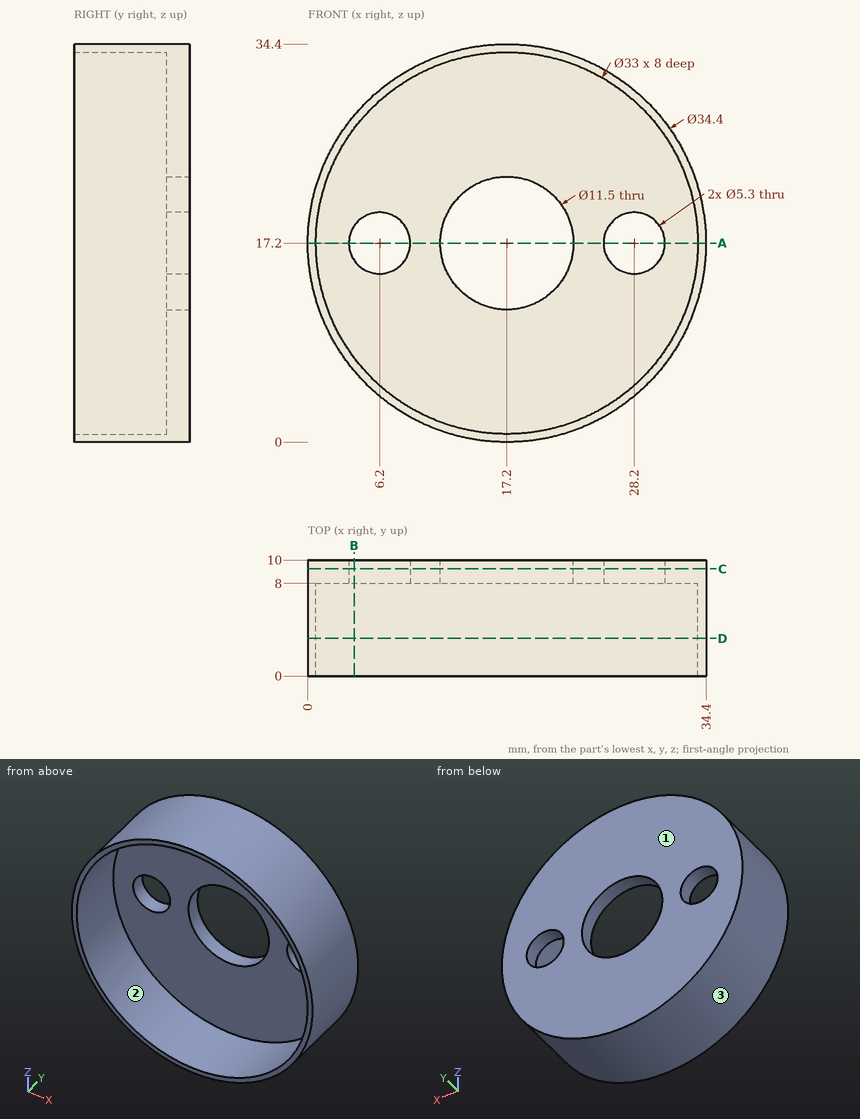
The figure shows three views and two pictorial views of one solid part (mm, origin at its lowest corner). Answer the questions. Give positions to 0.01 mm unless a question says otherwise; leave off trailing zeros. Order: outer loops, then holes, each group sorted by start corner. A loop starts at its lowest first (then second) coordinate and runs counter-clockwise, first axis right, second up. Notation, with made-up numbers: (34.25, 28) -> (70.25, 28) arc R28 ccw to (70.25, 62) -> close; hole circle Ø5 at (-10.75, 20.5). An arc over 180 degrees is marked (long way). Answer as a JSON object with one key per item and string values. Group by question number.
Item 1: The part is cut by section D-D on y = 3.25. Write down the section's boundary in (x, z), and give its area (3 significant figures).
Item 2: The part is cut by section C-C on y = 9.25. Write down the section's boundary in (x, z), and give its area (3 significant figures).
Item 3: The part is cut by section A-A on z = 17.2. Write down the section's boundary in (x, y).
Item 4: Flat-ended cylindrical pins translate along their axes: pin 1 (2 mm diameter, centred on x = 29, z = 8, fed in from -Y); pin 2 (6 mm diameter, centred on y = 6, z = 13, fed in from +X). Find the tip coordinate at first contact, or state that the pin passes through.
Item 5: The part is cut by section B-B on x = 4. Write down the section's boundary in (y, z).
Item 6: Determine the mould class of the marked faces 1, 2 and 3 for opening direction Z: pulls with the +Z half, pulls with the -Z half, needs draft (parallel to the pull), parting line crosses it, or undercut.
Item 7: Consider L1, parallel to X at y = 8.75, z = 17.2; L2, parallel to X at y = 6.5, z = 17.2; L3, parallel to Y at x = 27.5, z = 22. Determine where each line is inside the solid, lowest interval first. Write a range as from..to.
Result set:
{
 "1": {"outline": "circle Ø34.4 at (17.2, 17.2); hole circle Ø33 at (17.2, 17.2)", "area": "74.1 mm²"},
 "2": {"outline": "circle Ø34.4 at (17.2, 17.2); hole circle Ø5.3 at (6.2, 17.2); hole circle Ø11.5 at (17.2, 17.2); hole circle Ø5.3 at (28.2, 17.2)", "area": "781 mm²"},
 "3": {"outline": "(0, 0) -> (0.7, 0) -> (0.7, 8) -> (3.55, 8) -> (3.55, 10) -> (0, 10) -> close; (8.85, 8) -> (11.45, 8) -> (11.45, 10) -> (8.85, 10) -> close; (22.95, 8) -> (25.55, 8) -> (25.55, 10) -> (22.95, 10) -> close; (30.85, 8) -> (33.7, 8) -> (33.7, 0) -> (34.4, 0) -> (34.4, 10) -> (30.85, 10) -> close"},
 "4": {"pin 1": "y = 8", "pin 2": "x = 34.36"},
 "5": {"outline": "(0, 6.17) -> (10, 6.17) -> (10, 15.72) -> (8, 15.72) -> (8, 7.3) -> (0, 7.3) -> close; (0, 27.1) -> (8, 27.1) -> (8, 18.68) -> (10, 18.68) -> (10, 28.23) -> (0, 28.23) -> close"},
 "6": {"face 1": "needs draft", "face 2": "undercut", "face 3": "parting line crosses it"},
 "7": {"L1": "0..3.55, 8.85..11.45, 22.95..25.55, 30.85..34.4", "L2": "0..0.7, 33.7..34.4", "L3": "8..10"}
}
